Verification items for this drawing (mm, ordinates from the low corner). A direction names the side the tool comes from. Coordinates: 2 decimals unless noted, no trailing zeros. Write each loop counter-clockwise with the first axis right and the second up, starting at its lowest first coordinate (ties: lowest second). Pieces come first, ordered by that corner, then holes. Notation, with made-up numbers: (27.5, 22.5) -> (51.5, 22.5) arc R14 ccw to (51.5, 45.5) -> close; hole circle Ø8 at (-31.75, -30.75). An arc over 180 degrees is marked (long way). One line per item, written item: value. Start each with the question number.
1) Gauge pin test, flat ends, axial feed: P1, Ø4.5, axis at x = 47.5, z = 7.5, coming from the +Y side; P2, Ø3, axis at x = 56, z = 18.5, coming from the +Y side; P3, Ø5, axis at x = 41, y = 36, coming from the +Z side; P4, Ø1, axis at x = 18.5, y = 16.5, coming from the +Z side. Record the tip position at first contact, or that the pin passes through.
2) Sectioned sample at D-D on z = 36.5. Enter the section's corners in (x, y).
3) Scan lines: line 1 along X through (y, z) = (29, 33.5); line 2 along Z through (x, y) = (49, 22). Record each from-to range of solid material in increasing order. Write a range as [from, to].
4) Sectioned sample at C-C on y = 20. Enter the section's corners in (x, z), plus the area to 3 significant figures.
5) Set-up check for the marked faces 1, 2 and 3: record each of +Z, -Z, +X, -X, +Y, -Y from which the full face is reachable in a straight line by a thin tool's end or side.
6) Sectioned sample at A-A on z = 21. Enter the section's corners in (x, y), plus the area to 3 significant figures.
7) Sectioned sample at B-B on x = 56. Enter the section's corners in (y, z), plus the area to 3 significant figures.
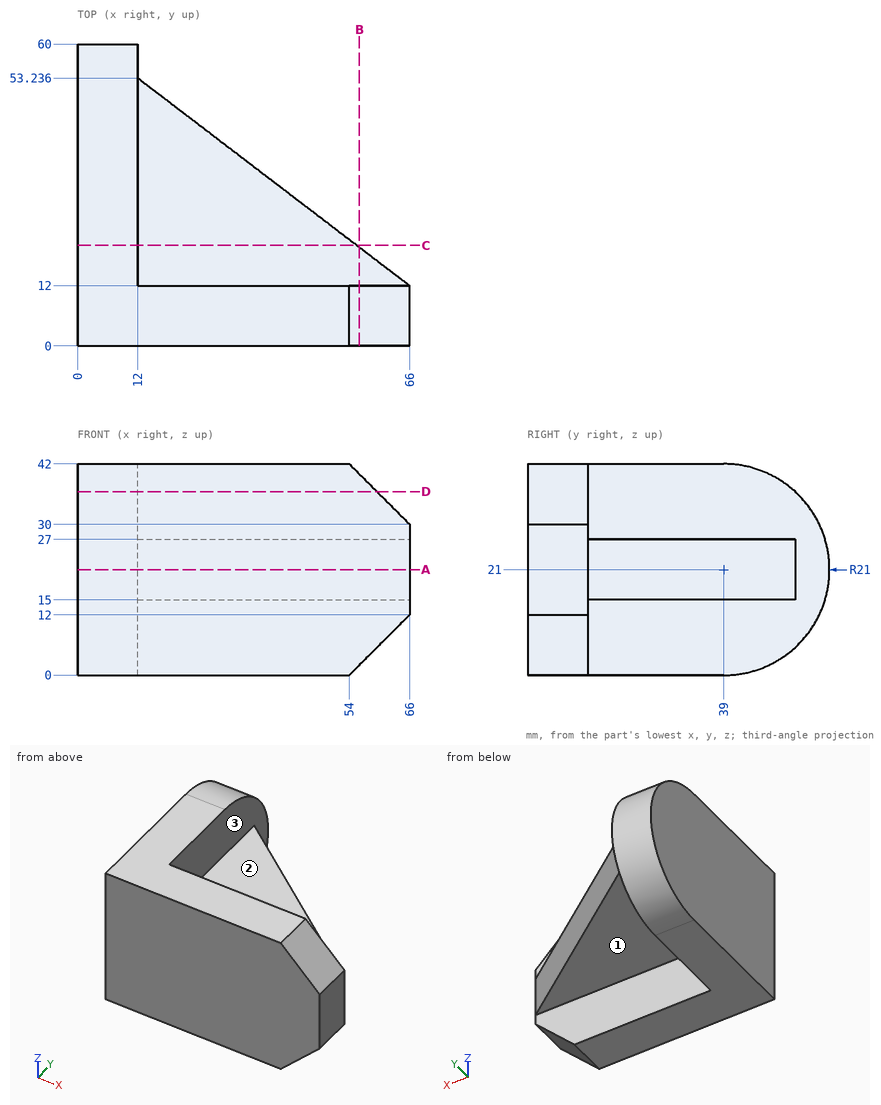
Answers:
1. P1: stops at y = 12
1. P2: stops at y = 20.78
1. P3: passes through
1. P4: stops at z = 27
2. outline: (0, 0) -> (59.5, 0) -> (59.5, 12) -> (12, 12) -> (12, 53.17) -> (0, 53.17) -> close
3. line 1: x = [0, 12]
3. line 2: z = [15, 27]
4. outline: (0, 0) -> (12, 0) -> (12, 15) -> (55.52, 15) -> (55.52, 27) -> (12, 27) -> (12, 42) -> (0, 42) -> close
4. area: 1,030 mm2
5. face 1: -Z, +X, +Y
5. face 2: +Z, +X, +Y
5. face 3: +X, +Y
6. outline: (0, 0) -> (66, 0) -> (66, 12) -> (12, 53.24) -> (12, 60) -> (0, 60) -> close
6. area: 2,480 mm2
7. outline: (0, 2) -> (12, 2) -> (12, 15) -> (19.64, 15) -> (19.64, 27) -> (12, 27) -> (12, 40) -> (0, 40) -> close
7. area: 548 mm2
